The model under review builds one solid part; all positions refer to its coordinate system, in mm. Face numbers are marked on the shaded views. A direction names the side the tool comes from. Round coordinates to 2 decimals unless told otherwise and drop trailing zeros. Loops run counter-clockwise (first coordinate to the right, second up) from the corner with the lowest first, then second, coordinate; pieces in that order, holes last. Notation, with made-up numbers: (-26.75, 24.5) -> (-19.75, 24.5) arc R19 cw to (-19.75, 28.5) -> close; hole circle Ø7 at (-34, 56). An arc over 180 degrees is marked (long way). Use a Markdown table: item, result. Add a question column.
1) Wall thickness on probe 1 along Y at (x, z) = (76.2, 17); probe 2 along Y at (x, z) = (-91.5, 9.5): over which ranges is each line inside the solid? List them lowest first.
2) Consider section D-D on z = 4. Give the boundary of the cut face in (x, y), plus the area to 3 significant figures.
3) Consider section A-A on x = 76.2. Give the boundary of the cut face in (y, z).
4) Mouldability with a two-part tool opening along Y and no side actions: class the marked faces 3, 4, 5 and 6 as released by +Y, released by -Y, zero draft, split by the parting line, or undercut.
5) For the marked faces 1 and 2, list the 3-axis set-ups (+Z, -Z, +X, -X, +Y, -Y) from which the entire face can be reached by the end or side of a thin tool; tool diameter is ignored.
6) Consider section C-C on z = 24. State how many separate pieces and enclosed holes the cut face has, plus the area to 3 significant figures.
from build123d import *

# Parameters (mm, degrees)
F0_W     = 304.8
F0_H     = 304.8
F0_R     = 19.1135
F1_DEPTH = 31.75
F3_DEPTH = 12.7
F4_R     = 6.35


with BuildPart() as f1:
    # F0 (on Top) → F1 (new body)
    with BuildSketch(Plane.XY):
        Rectangle(F0_W, F0_H)
        with Locations((-76.2, -76.2)):
            Circle(F0_R, mode=Mode.SUBTRACT)
        with Locations((76.2, -76.2)):
            Circle(F0_R, mode=Mode.SUBTRACT)
        with Locations((-76.2, 76.2)):
            Circle(F0_R, mode=Mode.SUBTRACT)
        with Locations((76.2, 76.2)):
            Circle(F0_R, mode=Mode.SUBTRACT)
    extrude(amount=F1_DEPTH)

    # F2 (on face) → F3 (cut)
    with BuildSketch(Plane.XY.offset(31.75)):
        with BuildLine():
            ThreePointArc((41.275, 34.925), (39.415128, 39.415128), (34.925, 41.275))
            Line((34.925, 41.275), (-34.925, 41.275))
            ThreePointArc((-34.925, 41.275), (-39.415128, 39.415128), (-41.275, 34.925))
            Line((-41.275, 34.925), (-41.275, -34.925))
            ThreePointArc((-41.275, -34.925), (-39.415128, -39.415128), (-34.925, -41.275))
            Line((-34.925, -41.275), (34.925, -41.275))
            ThreePointArc((34.925, -41.275), (39.415128, -39.415128), (41.275, -34.925))
            Line((41.275, -34.925), (41.275, 34.925))
        make_face()
    extrude(amount=-F3_DEPTH, mode=Mode.SUBTRACT)

    # F4
    f4_edges = [f1.edges().sort_by_distance(p)[0] for p in [
        (152.4, 152.4, 15.875),
        (152.4, -152.4, 15.875),
        (-152.4, 152.4, 15.875),
        (-152.4, -152.4, 15.875),
    ]]
    fillet(f4_edges, radius=F4_R)


solid = f1.part
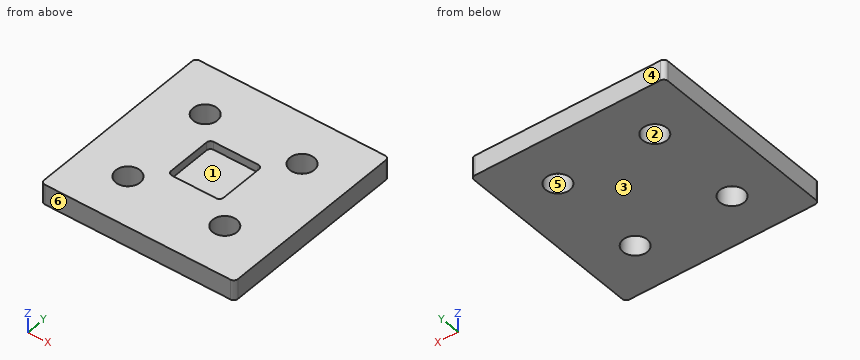
Result set:
| question | item | result |
|---|---|---|
| 1 | probe 1 | -152.4 to -95.31, -57.09 to 57.09, 95.31 to 152.4 |
| 1 | probe 2 | -152.4 to -87.66, -64.74 to 64.74, 87.66 to 152.4 |
| 2 | outline | (-152.4, -146.05) arc R6.35 ccw to (-146.05, -152.4) -> (146.05, -152.4) arc R6.35 ccw to (152.4, -146.05) -> (152.4, 146.05) arc R6.35 ccw to (146.05, 152.4) -> (-146.05, 152.4) arc R6.35 ccw to (-152.4, 146.05) -> close; hole circle Ø38.23 at (-76.2, -76.2); hole circle Ø38.23 at (-76.2, 76.2); hole circle Ø38.23 at (76.2, -76.2); hole circle Ø38.23 at (76.2, 76.2) |
| 2 | area | 88,300 mm2 |
| 3 | outline | (-152.4, 0) -> (-95.31, 0) -> (-95.31, 31.75) -> (-152.4, 31.75) -> close; (-57.09, 0) -> (57.09, 0) -> (57.09, 31.75) -> (-57.09, 31.75) -> close; (95.31, 0) -> (152.4, 0) -> (152.4, 31.75) -> (95.31, 31.75) -> close |
| 4 | face 3 | zero draft |
| 4 | face 4 | released by +Y |
| 4 | face 5 | undercut |
| 4 | face 6 | released by -Y |
| 5 | face 1 | +Z |
| 5 | face 2 | +Z, -Z |
| 6 | separate pieces | 1 |
| 6 | enclosed holes | 5 |
| 6 | area | 81,500 mm2 |
